Can you work these out from the model? Positions are in its coordinate system, mm. A direction names the side the tool comes from. Coordinates: 2 decimals unless noted, no trailing zeros. Order: outer loops, then holes, each group sorted by start corner. A loop starts at its lowest first (then second) coordinate and runs counter-clockwise, first axis right, second up. Notation, with made-up numbers: (-35.75, 73) -> (-10.75, 73) arc R29 ccw to (-10.75, 101) -> close; hole circle Ø8 at (57.25, -15.75). An arc over 180 degrees is marked (long way). Answer in a Markdown table with one row per item. Add a question column.
1. If I drill on line 1 along Y through (x, z) = (0, 6); line 2 along Z through (x, y) = (15.5, -5); line 3 along Y through (x, z) = (-7, 4.5), over which ranges is the centre line in solid material (lowest first)? Write a range as [from, to].
2. On a 3-axis mill with a long thin cutter (end or side, diameter ignored), from which of +Z, -Z, +X, -X, +Y, -Y can I reach the whole of each face in a straight line? I mean faces 1 (the face through (0, 0, 4.572)), 2 (the face through (-18.3, -16.5, 6.168)). Say none if no direction works.
3. Imagine slicing it at A-A on y = 0. Write out the boundary of the cut face in (x, z).
4. We'd pull the mould along X, two halves only. Please class faces 3 (the face through (18.7, -16.81, 5.842)), 4 (the face through (-5.506, -24.796, 5.216)), 5 (the face through (0, 0, 5.842)): pulls with the +X half, pulls with the -X half, needs draft (parallel to the pull), parting line crosses it, or undercut.
5. Imagine slicing it at C-C on z = 5.2. Write out the boundary of the cut face in (x, y), plus the area to 3 significant figures.
6. Will these pins go through, and if not, where does the flat tip stop? pin 1 (1 mm diameter, centred on x = -11.5, y = 4.5, fed in from +Z); pin 2 (15 mm diameter, centred on x = 7, y = 1, fed in from -Z).
from build123d import *

# Parameters (mm, degrees)
F0_W    = 24.3568923324
F0_H    = 1.27
F0_W_2  = 0.635
F0_W_3  = 0.4081076676
F0_H_2  = 0.3256250771
F0_H_3  = 0.3093749229
F2_SIZE = 0.127
F3_SIZE = 0.127
F4_SIZE = 0.127
F5_SIZE = 0.127


with BuildPart() as f1:
    # F0 (on Front) → F1 (revolve)
    with BuildSketch(Plane.XZ):
        with Locations((12.1784461662, 5.207)):
            Rectangle(F0_W, F0_H)
        with Locations((24.6743923324, 5.207)):
            Rectangle(F0_W_2, F0_H)
        with Locations((25.1959461662, 5.207)):
            Rectangle(F0_W_3, F0_H)
        with Locations((24.6743923324, 6.0048125385)):
            Rectangle(F0_W_2, F0_H_2)
        with Locations((24.6743923324, 4.4173125385)):
            Rectangle(F0_W_2, F0_H_3)
    revolve(axis=Axis((0, 0, 5.207), (0, 0, 1)))

    # F2
    f2_edges = [f1.edges().sort_by_distance(p)[0] for p in [
        (-24.991892, 0, 6.167625),
    ]]
    chamfer(f2_edges, length=F2_SIZE)

    # F3
    f3_edges = [f1.edges().sort_by_distance(p)[0] for p in [
        (-24.356892, 0, 6.167625),
    ]]
    chamfer(f3_edges, length=F3_SIZE)

    # F4
    f4_edges = [f1.edges().sort_by_distance(p)[0] for p in [
        (-24.991892, 0, 4.262625),
    ]]
    chamfer(f4_edges, length=F4_SIZE)

    # F5
    f5_edges = [f1.edges().sort_by_distance(p)[0] for p in [
        (-24.356892, 0, 4.262625),
    ]]
    chamfer(f5_edges, length=F5_SIZE)


solid = f1.part
Answers follow:
| question | item | result |
|---|---|---|
| 1 | line 1 | y = [-24.99, -24.36], [24.36, 24.99] |
| 1 | line 2 | z = [4.57, 5.84] |
| 1 | line 3 | y = [-23.99, -23.33], [23.33, 23.99] |
| 2 | face 1 | -Z |
| 2 | face 2 | +Z, +X, -X, +Y, -Y |
| 3 | outline | (-25.4, 4.57) -> (-24.99, 4.57) -> (-24.99, 4.39) -> (-24.86, 4.26) -> (-24.48, 4.26) -> (-24.36, 4.39) -> (-24.36, 4.57) -> (24.36, 4.57) -> (24.36, 4.39) -> (24.48, 4.26) -> (24.86, 4.26) -> (24.99, 4.39) -> (24.99, 4.57) -> (25.4, 4.57) -> (25.4, 5.84) -> (24.99, 5.84) -> (24.99, 6.04) -> (24.86, 6.17) -> (24.48, 6.17) -> (24.36, 6.04) -> (24.36, 5.84) -> (-24.36, 5.84) -> (-24.36, 6.04) -> (-24.48, 6.17) -> (-24.86, 6.17) -> (-24.99, 6.04) -> (-24.99, 5.84) -> (-25.4, 5.84) -> close |
| 4 | face 3 | needs draft |
| 4 | face 4 | parting line crosses it |
| 4 | face 5 | undercut |
| 5 | outline | circle Ø50.8 at (0, 0) |
| 5 | area | 2,030 mm² |
| 6 | pin 1 | stops at z = 5.84 |
| 6 | pin 2 | stops at z = 4.57 |
